from build123d import *

# Parameters (mm, degrees)
BOSS_EXTRUDE2_DEPTH = 3
SKETCH6_W           = 7.2
SKETCH6_H           = 3
BOSS_EXTRUDE3_DEPTH = 10.1
SKETCH8_R           = 1.4975
CUT_EXTRUDE3_DEPTH  = 45.922405323
SKETCH9_W           = 9
SKETCH9_H           = 9
BOSS_EXTRUDE4_DEPTH = 3
CHAMFER2_SIZE       = 3.464101615
CHAMFER2_SIZE_2     = 6
CHAMFER2_SIZE_3     = 3.099985421


# Read off the part's stored shape, not the designer's step: Mirror10
with BuildPart() as part:
    # Sketch4 → Boss-Extrude2 (new body)
    with BuildSketch(Plane(origin=(10.1, 0, 0), x_dir=(0, 0, -1), z_dir=(1, 0, 0))):
        Polygon((0, 0), (20.3, 0), (20.3, 3), (27.7, 29.85), (27.7, 32.85), (20.5, 32.85), (12.273184358, 3), (0, 3), align=None)
        Polygon((22.785036556, 29.85), (15.385036556, 3), (17.188147801, 3), (24.588147801, 29.85), align=None, mode=Mode.SUBTRACT)
    boss_extrude2 = extrude(amount=BOSS_EXTRUDE2_DEPTH)

    # Sketch6 → Boss-Extrude3 (add)
    with BuildSketch(Plane.ZY.offset(-10.1)):
        with Locations((-24.1, 31.35)):
            Rectangle(SKETCH6_W, SKETCH6_H)
    boss_extrude3 = extrude(amount=BOSS_EXTRUDE3_DEPTH)

    # Sketch8 → Cut-Extrude3 (cut, through all)
    with BuildSketch(Plane(origin=(0, 32.85, 0), x_dir=(1, 0, 0), z_dir=(0, 1, 0))):
        with Locations(Location((5, 24.3, 0), (0, 0, 270))):
            Circle(SKETCH8_R)
    cut_extrude3 = extrude(amount=-CUT_EXTRUDE3_DEPTH, mode=Mode.SUBTRACT)

    # Sketch9 → Boss-Extrude4 (add)
    with BuildSketch(Plane.XZ):
        with Locations((14.6, -21.8)):
            Rectangle(SKETCH9_W, SKETCH9_H)
    boss_extrude4 = extrude(amount=-BOSS_EXTRUDE4_DEPTH)

    # Mirror9: Boss-Extrude2, Boss-Extrude3, Cut-Extrude3, Boss-Extrude4 across plane
    add(boss_extrude2.mirror(Plane(origin=(0, 0, 0), x_dir=(0, 0, 1), z_dir=(1, 0, 0))))
    add(boss_extrude3.mirror(Plane(origin=(0, 0, 0), x_dir=(0, 0, 1), z_dir=(1, 0, 0))))
    add(cut_extrude3.mirror(Plane(origin=(0, 0, 0), x_dir=(0, 0, 1), z_dir=(1, 0, 0))), mode=Mode.SUBTRACT)
    add(boss_extrude4.mirror(Plane(origin=(0, 0, 0), x_dir=(0, 0, 1), z_dir=(1, 0, 0))))

    # Mirror10: part across plane


with BuildPart() as part_1:
    add(part.part)
    add(part.part.mirror(Plane.XY))

    # Chamfer2
    # the kernel refuses this chamfer: 6, 3.464101615, 3.099985421 mm, written as the material it adds along each edge
    with BuildSketch(Plane(origin=(-13.1, 3, 17.3), x_dir=(-0.9983227437537925, -0.05789386240267071, 0), z_dir=(0, 0, 1))) as chamfer2_piece_1_section:
        Polygon((CHAMFER2_SIZE * 0.998322743793, -CHAMFER2_SIZE * 0.057893862405), (-CHAMFER2_SIZE_2 * 0.0578938624027, -CHAMFER2_SIZE_2 * 0.998322743754), (0, 0), align=None)
    chamfer2_piece_1 = extrude(amount=18.522514528, mode=Mode.PRIVATE)
    chamfer2_piece_1 = split(chamfer2_piece_1, bisect_by=Plane(origin=(-14.207429755, 4.623813367, 20.747531431), z_dir=(0, 0.2656988795293601, -0.9640560696436917)), keep=Keep.TOP, mode=Mode.PRIVATE)
    chamfer2_piece_1 = split(chamfer2_piece_1, bisect_by=Plane(origin=(-14.207429755, 5.420910005, 17.855363222), z_dir=(0, -0.26569887952935983, 0.9640560696436918)), keep=Keep.TOP, mode=Mode.PRIVATE)
    add(chamfer2_piece_1)
    with BuildSketch(Plane(origin=(-13.1, 3, -17.3), x_dir=(-0.9983227437537925, -0.05789386240267071, 0), z_dir=(0, 0, -1))) as chamfer2_piece_2_section:
        Polygon((CHAMFER2_SIZE * 0.998322743793, CHAMFER2_SIZE * 0.057893862405), (-CHAMFER2_SIZE_2 * 0.0578938624027, CHAMFER2_SIZE_2 * 0.998322743754), (0, 0), align=None)
    chamfer2_piece_2 = extrude(amount=18.522514528, mode=Mode.PRIVATE)
    chamfer2_piece_2 = split(chamfer2_piece_2, bisect_by=Plane(origin=(-14.207429755, 5.420910005, -17.855363222), z_dir=(0, -0.26569887952935983, -0.9640560696436918)), keep=Keep.TOP, mode=Mode.PRIVATE)
    chamfer2_piece_2 = split(chamfer2_piece_2, bisect_by=Plane(origin=(-14.207429755, 4.623813367, -20.747531431), z_dir=(0, 0.2656988795293601, 0.9640560696436917)), keep=Keep.TOP, mode=Mode.PRIVATE)
    add(chamfer2_piece_2)
    with BuildSketch(Plane(origin=(-10.1, 3, 20.3), x_dir=(0, -0.07329167604498149, 0.997310548536672), z_dir=(-1, 0, 0)), Plane(origin=(10.1, 3, -20.3), x_dir=(0, -0.07329167604498149, -0.997310548536672), z_dir=(1, 0, 0))) as chamfer2_piece_3:
        Polygon((CHAMFER2_SIZE_3 * 0.997310548488, CHAMFER2_SIZE_3 * 0.0732916760414), (CHAMFER2_SIZE_2 * 0.194327010143, CHAMFER2_SIZE_2 * 0.98093680384), (0, 0), align=None)
    extrude(amount=3)
    with BuildSketch(Plane(origin=(13.1, 3, 35.822514528), x_dir=(0.9983227437537925, -0.05789386240267071, 0), z_dir=(0, 0, -1))) as chamfer2_piece_4_section:
        Polygon((CHAMFER2_SIZE * 0.998322743793, -CHAMFER2_SIZE * 0.057893862405), (-CHAMFER2_SIZE_2 * 0.0578938624027, -CHAMFER2_SIZE_2 * 0.998322743754), (0, 0), align=None)
    chamfer2_piece_4 = extrude(amount=18.522514528, mode=Mode.PRIVATE)
    chamfer2_piece_4 = split(chamfer2_piece_4, bisect_by=Plane(origin=(14.207429755, 4.623813367, 20.747531431), z_dir=(0, 0.2656988795293601, -0.9640560696436917)), keep=Keep.TOP, mode=Mode.PRIVATE)
    chamfer2_piece_4 = split(chamfer2_piece_4, bisect_by=Plane(origin=(14.207429755, 5.420910005, 17.855363222), z_dir=(0, -0.26569887952935983, 0.9640560696436918)), keep=Keep.TOP, mode=Mode.PRIVATE)
    add(chamfer2_piece_4)
    with BuildSketch(Plane(origin=(13.1, 3, -35.822514528), x_dir=(0.9983227437537925, -0.05789386240267071, 0), z_dir=(0, 0, 1))) as chamfer2_piece_5_section:
        Polygon((CHAMFER2_SIZE * 0.998322743793, CHAMFER2_SIZE * 0.057893862405), (-CHAMFER2_SIZE_2 * 0.0578938624027, CHAMFER2_SIZE_2 * 0.998322743754), (0, 0), align=None)
    chamfer2_piece_5 = extrude(amount=18.522514528, mode=Mode.PRIVATE)
    chamfer2_piece_5 = split(chamfer2_piece_5, bisect_by=Plane(origin=(14.207429755, 4.623813367, -20.747531431), z_dir=(0, 0.2656988795293601, 0.9640560696436917)), keep=Keep.TOP, mode=Mode.PRIVATE)
    chamfer2_piece_5 = split(chamfer2_piece_5, bisect_by=Plane(origin=(14.207429755, 5.420910005, -17.855363222), z_dir=(0, -0.26569887952935983, -0.9640560696436918)), keep=Keep.TOP, mode=Mode.PRIVATE)
    add(chamfer2_piece_5)
    with BuildSketch(Plane(origin=(10.1, 3, 20.3), x_dir=(0, 0.9690111038190681, 0.24701716676245647), z_dir=(1, 0, 0))) as chamfer2_piece_6:
        Polygon((CHAMFER2_SIZE_2 * 0.999813220622, CHAMFER2_SIZE_2 * 0.0193267656127), (CHAMFER2_SIZE_3 * 0.247017166751, CHAMFER2_SIZE_3 * 0.969011103772), (0, 0), align=None)
    extrude(amount=3)
    with BuildSketch(Plane(origin=(-10.1, 3, -20.3), x_dir=(0, -0.07329167604498149, -0.997310548536672), z_dir=(-1, 0, 0))) as chamfer2_piece_7:
        Polygon((CHAMFER2_SIZE_3 * 0.997310548488, -CHAMFER2_SIZE_3 * 0.0732916760414), (CHAMFER2_SIZE_2 * 0.194327010143, -CHAMFER2_SIZE_2 * 0.98093680384), (0, 0), align=None)
    extrude(amount=3)
    with BuildSketch(Plane(origin=(-13.1, 3, 17.3), x_dir=(-0.9983227437537925, -0.05789386240267071, 0), z_dir=(0, 0, 1))) as chamfer2_piece_8a_section:
        Polygon((CHAMFER2_SIZE * 0.998322743793, -CHAMFER2_SIZE * 0.057893862405), (-CHAMFER2_SIZE_2 * 0.0578938624027, -CHAMFER2_SIZE_2 * 0.998322743754), (0, 0), align=None)
    chamfer2_piece_8a = extrude(amount=18.522514528, mode=Mode.PRIVATE)
    chamfer2_piece_8a = split(chamfer2_piece_8a, bisect_by=Plane(origin=(-14.24841762, 4.892203589, 26.3), z_dir=(0, 0, -1)), keep=Keep.TOP, mode=Mode.PRIVATE)
    chamfer2_piece_8a = split(chamfer2_piece_8a, bisect_by=Plane(origin=(-14.24841762, 5.593858539, 21.014880938), z_dir=(0, -0.2656988795293601, 0.9640560696436917)), keep=Keep.TOP, mode=Mode.PRIVATE)
    with BuildSketch(Plane(origin=(-10.1, 3, 20.3), x_dir=(0, -0.07329167604498149, 0.997310548536672), z_dir=(-1, 0, 0))) as chamfer2_piece_8b_section:
        Polygon((CHAMFER2_SIZE_3 * 0.997310548488, CHAMFER2_SIZE_3 * 0.0732916760414), (CHAMFER2_SIZE_2 * 0.194327010143, CHAMFER2_SIZE_2 * 0.98093680384), (0, 0), align=None)
    chamfer2_piece_8b = extrude(amount=18.522514528, mode=Mode.PRIVATE)
    chamfer2_piece_8b = split(chamfer2_piece_8b, bisect_by=Plane(origin=(-19.1, 4.952235463, 21.823438055), z_dir=(1, 0, 0)), keep=Keep.TOP, mode=Mode.PRIVATE)
    chamfer2_piece_8b = split(chamfer2_piece_8b, bisect_by=Plane(origin=(-13.1, 4.952235463, 21.823438055), z_dir=(-1, 0, 0)), keep=Keep.TOP, mode=Mode.PRIVATE)
    chamfer2_piece_8 = chamfer2_piece_8a & chamfer2_piece_8b
    add(chamfer2_piece_8)
    with BuildSketch(Plane(origin=(-13.1, 3, -17.3), x_dir=(-0.9983227437537925, -0.05789386240267071, 0), z_dir=(0, 0, -1))) as chamfer2_piece_9a_section:
        Polygon((CHAMFER2_SIZE * 0.998322743793, CHAMFER2_SIZE * 0.057893862405), (-CHAMFER2_SIZE_2 * 0.0578938624027, CHAMFER2_SIZE_2 * 0.998322743754), (0, 0), align=None)
    chamfer2_piece_9a = extrude(amount=18.522514528, mode=Mode.PRIVATE)
    chamfer2_piece_9a = split(chamfer2_piece_9a, bisect_by=Plane(origin=(-14.24841762, 4.892203589, -26.3), z_dir=(0, 0, 1)), keep=Keep.TOP, mode=Mode.PRIVATE)
    chamfer2_piece_9a = split(chamfer2_piece_9a, bisect_by=Plane(origin=(-14.24841762, 5.593858539, -21.014880938), z_dir=(0, -0.2656988795293601, -0.9640560696436917)), keep=Keep.TOP, mode=Mode.PRIVATE)
    with BuildSketch(Plane(origin=(-10.1, 3, -20.3), x_dir=(0, -0.07329167604498149, -0.997310548536672), z_dir=(-1, 0, 0))) as chamfer2_piece_9b_section:
        Polygon((CHAMFER2_SIZE_3 * 0.997310548488, -CHAMFER2_SIZE_3 * 0.0732916760414), (CHAMFER2_SIZE_2 * 0.194327010143, -CHAMFER2_SIZE_2 * 0.98093680384), (0, 0), align=None)
    chamfer2_piece_9b = extrude(amount=18.522514528, mode=Mode.PRIVATE)
    chamfer2_piece_9b = split(chamfer2_piece_9b, bisect_by=Plane(origin=(-19.1, 4.952235463, -21.823438055), z_dir=(1, 0, 0)), keep=Keep.TOP, mode=Mode.PRIVATE)
    chamfer2_piece_9b = split(chamfer2_piece_9b, bisect_by=Plane(origin=(-13.1, 4.952235463, -21.823438055), z_dir=(-1, 0, 0)), keep=Keep.TOP, mode=Mode.PRIVATE)
    chamfer2_piece_9 = chamfer2_piece_9a & chamfer2_piece_9b
    add(chamfer2_piece_9)
    with BuildSketch(Plane(origin=(10.1, 3, 20.3), x_dir=(0, 0.9690111038190681, 0.24701716676245647), z_dir=(1, 0, 0))) as chamfer2_piece_10a_section:
        Polygon((CHAMFER2_SIZE_2 * 0.999813220622, CHAMFER2_SIZE_2 * 0.0193267656127), (CHAMFER2_SIZE_3 * 0.247017166751, CHAMFER2_SIZE_3 * 0.969011103772), (0, 0), align=None)
    chamfer2_piece_10a = extrude(amount=18.522514528, mode=Mode.PRIVATE)
    chamfer2_piece_10a = split(chamfer2_piece_10a, bisect_by=Plane(origin=(13.1, 4.952235463, 21.823438055), z_dir=(1, 0, 0)), keep=Keep.TOP, mode=Mode.PRIVATE)
    chamfer2_piece_10a = split(chamfer2_piece_10a, bisect_by=Plane(origin=(19.1, 4.952235463, 21.823438055), z_dir=(-1, 0, 0)), keep=Keep.TOP, mode=Mode.PRIVATE)
    with BuildSketch(Plane(origin=(13.1, 3, 35.822514528), x_dir=(0.9983227437537925, -0.05789386240267071, 0), z_dir=(0, 0, -1))) as chamfer2_piece_10b_section:
        Polygon((CHAMFER2_SIZE * 0.998322743793, -CHAMFER2_SIZE * 0.057893862405), (-CHAMFER2_SIZE_2 * 0.0578938624027, -CHAMFER2_SIZE_2 * 0.998322743754), (0, 0), align=None)
    chamfer2_piece_10b = extrude(amount=18.522514528, mode=Mode.PRIVATE)
    chamfer2_piece_10b = split(chamfer2_piece_10b, bisect_by=Plane(origin=(14.24841762, 5.593858539, 21.014880938), z_dir=(0, -0.2656988795293601, 0.9640560696436917)), keep=Keep.TOP, mode=Mode.PRIVATE)
    chamfer2_piece_10b = split(chamfer2_piece_10b, bisect_by=Plane(origin=(14.24841762, 4.892203589, 26.3), z_dir=(0, 0, -1)), keep=Keep.TOP, mode=Mode.PRIVATE)
    chamfer2_piece_10 = chamfer2_piece_10a & chamfer2_piece_10b
    add(chamfer2_piece_10)
    with BuildSketch(Plane(origin=(13.1, 3, -35.822514528), x_dir=(0.9983227437537925, -0.05789386240267071, 0), z_dir=(0, 0, 1))) as chamfer2_piece_11a_section:
        Polygon((CHAMFER2_SIZE * 0.998322743793, CHAMFER2_SIZE * 0.057893862405), (-CHAMFER2_SIZE_2 * 0.0578938624027, CHAMFER2_SIZE_2 * 0.998322743754), (0, 0), align=None)
    chamfer2_piece_11a = extrude(amount=18.522514528, mode=Mode.PRIVATE)
    chamfer2_piece_11a = split(chamfer2_piece_11a, bisect_by=Plane(origin=(14.24841762, 4.892203589, -26.3), z_dir=(0, 0, 1)), keep=Keep.TOP, mode=Mode.PRIVATE)
    chamfer2_piece_11a = split(chamfer2_piece_11a, bisect_by=Plane(origin=(14.24841762, 5.593858539, -21.014880938), z_dir=(0, -0.2656988795293601, -0.9640560696436917)), keep=Keep.TOP, mode=Mode.PRIVATE)
    with BuildSketch(Plane(origin=(10.1, 3, -20.3), x_dir=(0, -0.07329167604498149, -0.997310548536672), z_dir=(1, 0, 0))) as chamfer2_piece_11b_section:
        Polygon((CHAMFER2_SIZE_3 * 0.997310548488, CHAMFER2_SIZE_3 * 0.0732916760414), (CHAMFER2_SIZE_2 * 0.194327010143, CHAMFER2_SIZE_2 * 0.98093680384), (0, 0), align=None)
    chamfer2_piece_11b = extrude(amount=18.522514528, mode=Mode.PRIVATE)
    chamfer2_piece_11b = split(chamfer2_piece_11b, bisect_by=Plane(origin=(19.1, 4.952235463, -21.823438055), z_dir=(-1, 0, 0)), keep=Keep.TOP, mode=Mode.PRIVATE)
    chamfer2_piece_11b = split(chamfer2_piece_11b, bisect_by=Plane(origin=(13.1, 4.952235463, -21.823438055), z_dir=(1, 0, 0)), keep=Keep.TOP, mode=Mode.PRIVATE)
    chamfer2_piece_11 = chamfer2_piece_11a & chamfer2_piece_11b
    add(chamfer2_piece_11)


solid = part_1.part
Input: part model. Units: mm. Frame: model coordinates. A direction names the side the tool comes from. Round coordinates to 2 decimals unless told otherwise and drop trailing zeros. Order: outer loops, then holes, each group sorted by start corner. A loop starts at its lowest first (then second) coordinate and runs counter-clockwise, first axis right, second up. Notation, with made-up numbers: (72, 36.25) - (89, 36.25) arc R8 ccw to (89, 51.25) - close; hole circle Ø6 at (-9, -24). An arc over 180 degrees is marked (long way). Answer as a JSON object with one key per item and string values. Group by question number.
(1) Draft query along Z for faces 1 (the face through (-11.579, 18.134, 16.444)), 2 (the face through (-15, 1, -26.3)), 3 (the face through (-11.579, 16.613, -19.137)), 4 (the face through (0, 32.85, 24)). Return one class per face: released by +Z, released by -Z, zero draft, split by the parting line, or undercut.
(2) Cut plane D-D (z = -18). Return loops of the section in (x, y).
(3) Pin query (flat end, axial travel): P1, Ø1.7, axis at x = 17, y = 2, coming from the -Z side; P2, Ø1.5, axis at x = -11, y = 15, coming from the +Z side; P3, Ø5, axis at x = -5, z = -24.3, coming from the -Y side. Return the tip coordinate at first contact, or that it passes through.
(4) Cut plane B-B (x = -11.5). Return loops of the section in (y, z), then the cut area to 3 significant figures.
(5) Reachability of faces 5 (the face through (0, 31, -20.5)), 6 (the face through (-11.684, 19.465, 24.838)), 7 (the face through (-16, 3, -24)) from +Z, -Z, +X, -X, +Y, -Y: full face, straight path, thin tool, end or side. Return the list, or none.
(6) Cut plane C-C (z = 0.5). Return loops of the section in (x, y).
(7) Material intervals for probe 1 along Z at (x, y) = (-5, 31.75); probe 2 along X at (y, z) = (4, 14); probe 3 along X at (y, z) = (30, -24), sorted ascending. Write a range as from..to.
(8) Cut plane A-A (x = 5). Return loops of the section in (y, z).
Here are the results:
{
 "1": {"face 1": "undercut", "face 2": "released by -Z", "face 3": "undercut", "face 4": "zero draft"},
 "2": {"outline": "(-19.1, 0) - (-10.1, 0) - (-10.1, 5.95) - (-14.86, 5.95) - (-16.56, 3) - (-19.1, 3) - close; (-13.1, 12.49) - (-10.1, 12.49) - (-10.1, 23.78) - (-13.1, 23.78) - close; (10.1, 0) - (19.1, 0) - (19.1, 3) - (16.56, 3) - (14.86, 5.95) - (10.1, 5.95) - close; (10.1, 12.49) - (13.1, 12.49) - (13.1, 23.78) - (10.1, 23.78) - close"},
 "3": {"P1": "stops at z = -26.3", "P2": "stops at z = 23.81", "P3": "stops at y = 29.85"},
 "4": {"outline": "(0, -26.3) - (3, -26.3) - (3, -23.4) - (8.78, -21.89) - (29.85, -27.7) - (32.85, -27.7) - (32.85, -20.5) - (3, -12.27) - (3, 12.27) - (32.85, 20.5) - (32.85, 27.7) - (29.85, 27.7) - (8.78, 21.89) - (3, 23.4) - (3, 26.3) - (0, 26.3) - close; hole (3, -17.19) - (29.85, -24.59) - (29.85, -22.79) - (3, -15.39) - close; hole (3, 15.39) - (29.85, 22.79) - (29.85, 24.59) - (3, 17.19) - close", "area": "556 mm^2"},
 "5": {"face 5": "+Y, -Y", "face 6": "+Z, +X, -X", "face 7": "-Z, -X"},
 "6": {"outline": "(-13.1, 0) - (-10.1, 0) - (-10.1, 3) - (-13.1, 3) - close; (10.1, 0) - (13.1, 0) - (13.1, 3) - (10.1, 3) - close"},
 "7": {"probe 1": "z = -27.7..-25.8, -22.8..-20.5, 20.5..22.8, 25.8..27.7", "probe 2": "x = -13.1..-10.1, 10.1..13.1", "probe 3": "x = -13.1..-6.47, -3.53..3.53, 6.47..13.1"},
 "8": {"outline": "(29.85, -27.7) - (32.85, -27.7) - (32.85, -25.8) - (29.85, -25.8) - close; (29.85, -22.8) - (32.85, -22.8) - (32.85, -20.5) - (29.85, -20.5) - close; (29.85, 20.5) - (32.85, 20.5) - (32.85, 22.8) - (29.85, 22.8) - close; (29.85, 25.8) - (32.85, 25.8) - (32.85, 27.7) - (29.85, 27.7) - close"}
}
